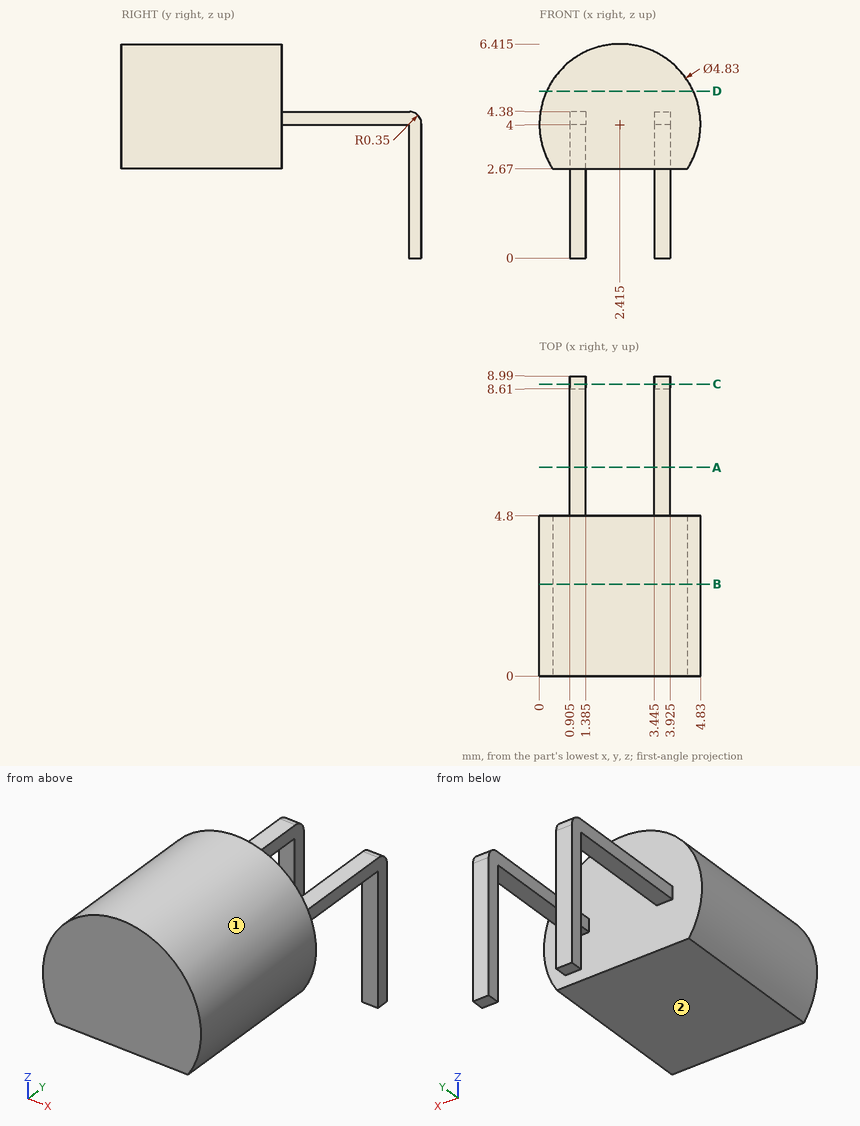
Here's the drawing with two shaded views (mm, measured from the low corner). I have some questions. A direction names the side the tool comes from. Give positions to 0.01 mm unless a question says otherwise; leave off trailing zeros. Loops run counter-clockwise (first coordinate to the right, second up) from the corner with the lowest first, then second, coordinate; pieces in that order, holes last. Notation, with made-up numbers: M 77,-2.5 L 132,-2.5 A24 ccw 132,32.5 Z; hole C 26,35.5 d7. An arc over 180 degrees is marked long. One line per item, written item: value. Start each with the question number.
1) If we section it at D-D, the plane z = 5: Write out the boundary of the cut face in (x, y).
2) If we section it at C-C, the plane y = 8.75: Write out the boundary of the cut face in (x, z) (3 decimals), and give its area (3 significant figures).
3) On a 3-axis mill with a long thin cutter (end or side, diameter ignored), from which of +Z, -Z, +X, -X, +Y, -Y can I reach the whole of each face in a straight line? I mean the marked faces 1 and 2. Say none if no direction works.
4) If we section it at A-A, the plane y = 6.25: Write out the boundary of the cut face in (x, z) (3 decimals), and give its area (3 significant figures).
5) I'm going to push flat-ended pins straight in: pin 1 (0.5 mm diameter, centred on x = 1, y = 7, fed in from +Z); pin 2 (0.5 mm diameter, centred on x = 1, z = 2, fed in from -Y); pin 3 (1 mm diameter, centred on x = 1.5, y = 2, fed in from +Z). Where does each tip first touch, or does it pass through?
6) If we section it at B-B, the plane y = 2.75: Write out the boundary of the cut face in (x, z) (3 decimals), and give its area (3 significant figures).
7) If I drill on line 1 (Y direction, x = 2.5, z = 3.5); line 2 (Z direction, x = 4.05, y = 1); line 3 (Z direction, x = 2.9, y = 2.5), over which ranges is the centre line in solid material (lowest first)? Write a range as [from, to].
Completed:
1. outline: M 0.22,0 L 4.61,0 L 4.61,4.8 L 0.22,4.8 Z
2. outline: M 0.905,0 L 1.385,0 L 1.385,4.362 L 0.905,4.362 Z; M 3.445,0 L 3.925,0 L 3.925,4.362 L 3.445,4.362 Z
2. area: 4.19 mm^2
3. face 1: +Y, -Y
3. face 2: -Z, +X, -X, -Y
4. outline: M 0.905,4 L 1.385,4 L 1.385,4.38 L 0.905,4.38 Z; M 3.445,4 L 3.925,4 L 3.925,4.38 L 3.445,4.38 Z
4. area: 0.365 mm^2
5. pin 1: stops at z = 4.38
5. pin 2: stops at y = 8.61
5. pin 3: stops at z = 6.38
6. outline: M 0.399,2.67 L 4.431,2.67 A2.415 ccw long Z
6. area: 15.2 mm^2
7. line 1: y = [0, 4.8]
7. line 2: z = [2.67, 5.78]
7. line 3: z = [2.67, 6.37]
